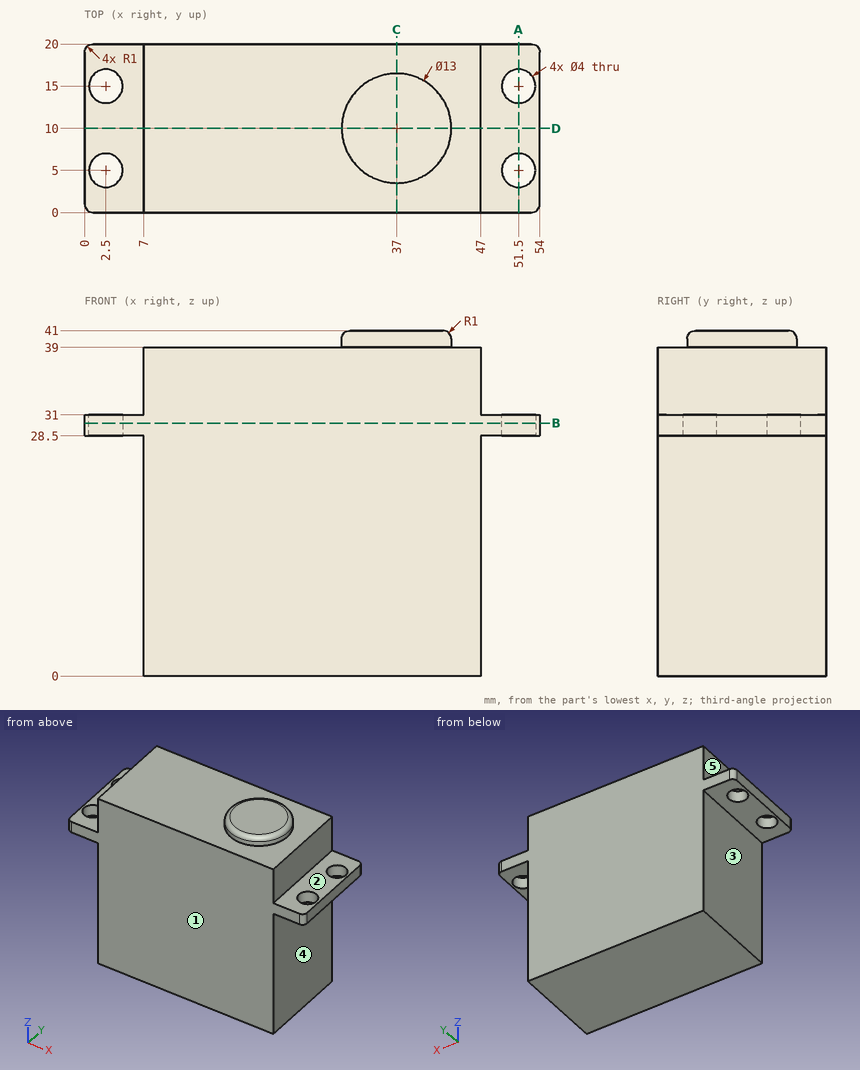
For this review, use the dimensioned drawing (mm, ordinates from the lowest corner) and the shaded views. A direction names the side the tool comes from. Round coordinates to 2 decimals unless told otherwise and drop trailing zeros. Write each loop counter-clockwise with the first axis right and the second up, starting at its lowest first coordinate (ties: lowest second). Pieces come first, ordered by that corner, then holes. Notation, with made-up numbers: (14.5, 1.5) -> (47.5, 1.5) arc R29 cw to (47.5, 34.5) -> close; hole circle Ø11 at (26, 8). An arc over 180 degrees is marked (long way). Use CSV: the item, a comma, the result in double quotes.
(1) Consider section B-B, the plane z = 30. Give the boundary of the cut face in (x, y).
Computed values:
outline,"(0, 1) arc R1 ccw to (1, 0) -> (53, 0) arc R1 ccw to (54, 1) -> (54, 19) arc R1 ccw to (53, 20) -> (1, 20) arc R1 ccw to (0, 19) -> close; hole circle Ø4 at (2.5, 5); hole circle Ø4 at (2.5, 15); hole circle Ø4 at (51.5, 5); hole circle Ø4 at (51.5, 15)"
(2) Consider section D-D, the plane y = 10. Give the boundary of the cut face in (x, z).
Computed values:
outline,"(0, 28.5) -> (7, 28.5) -> (7, 0) -> (47, 0) -> (47, 28.5) -> (54, 28.5) -> (54, 31) -> (47, 31) -> (47, 39) -> (43.5, 39) -> (43.5, 40) arc R1 ccw to (42.5, 41) -> (31.5, 41) arc R1 ccw to (30.5, 40) -> (30.5, 39) -> (7, 39) -> (7, 31) -> (0, 31) -> close"
(3) For the marked faces 1, 2, 3, 4 and 5, list the 3-axis set-ups (+Z, -Z, +X, -X, +Y, -Y) from which the entire face can be reached by the end or side of a thin tool; tool diameter is ignored.
Computed values:
face 1,"+Z, -Z, +X, -X, -Y"
face 2,"+Z, +X, +Y, -Y"
face 3,"-Z, -X, +Y, -Y"
face 4,"-Z, +X, +Y, -Y"
face 5,"+Z, -X, +Y, -Y"
(4) Clearance check with flat-ended pins moving along their axes: P1, Ø6, axis at x = 38.5, z = 29.5, coming from the -Y side; P2, Ø5, axis at y = 7, z = 22, coming from the -X side; P3, Ø2, axis at y = 5.5, z = 5.5, coming from the +X side; P4, Ø3, axis at x = 2.5, y = 15, coming from the +Z side. State where each tip first meets the part, or that it passes through.
Computed values:
P1,"y = 0"
P2,"x = 7"
P3,"x = 47"
P4,"through"
(5) Consider section A-A, the plane x = 51.5. Give the boundary of the cut face in (y, z).
Computed values:
outline,"(0, 28.5) -> (3, 28.5) -> (3, 31) -> (0, 31) -> close; (7, 28.5) -> (13, 28.5) -> (13, 31) -> (7, 31) -> close; (17, 28.5) -> (20, 28.5) -> (20, 31) -> (17, 31) -> close"
(6) To check wall thickness, follow L1, parallel to Y at x = 2.5, z = 29.9; L2, parallel to Z at x = 3.5, y = 18.75; L3, parallel to Z at x = 41, y = 4. State the ranges of each line that lie inside material, in increasing order. Write a range as [from, to].
Computed values:
L1,"[0, 3], [7, 13], [17, 20]"
L2,"[28.5, 31]"
L3,"[0, 39]"
(7) Consider section C-C, the plane x = 37. Give the boundary of the cut face in (y, z).
Computed values:
outline,"(0, 0) -> (20, 0) -> (20, 39) -> (16.5, 39) -> (16.5, 40) arc R1 ccw to (15.5, 41) -> (4.5, 41) arc R1 ccw to (3.5, 40) -> (3.5, 39) -> (0, 39) -> close"
